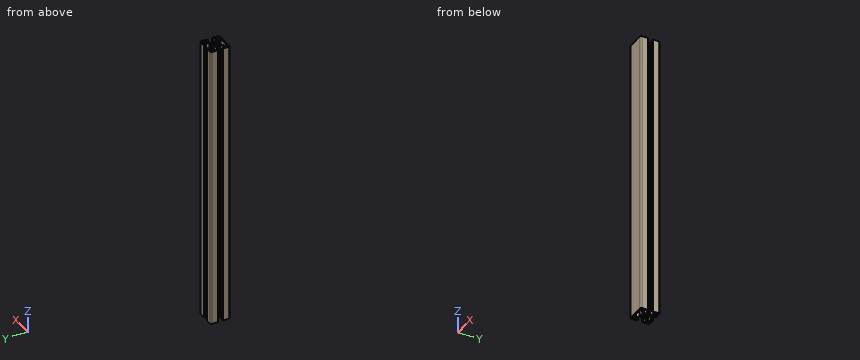
from build123d import *

# Parameters (mm, degrees)
ESTRUSIONE_ESTRUSIONE1_DEPTH = 450


with BuildPart() as part:
    # Schizzo1 → Estrusione-Estrusione1 (new body)
    with BuildSketch(Plane(origin=(0, 0, -450), x_dir=(-1, 0, 0), z_dir=(0, 0, -1))):
        with BuildLine():
            Line((-15, -4), (-15, -13))
            ThreePointArc((-15, -13), (-14.414213562, -14.414213562), (-13, -15))
            Line((-13, -15), (13, -15))
            ThreePointArc((13, -15), (14.414213562, -14.414213562), (15, -13))
            Line((15, -13), (15, -4))
            Line((15, -4), (13, -4))
            Line((13, -4), (13, -8.25))
            Line((13, -8.25), (9.664213562, -8.25))
            add(Edge.make_bspline(
                [(9.664213562, -8.25), (8.442809042, -7.028595479), (7.221404521, -5.807190958), (6, -4.585786438)],
                knots=[0, 0, 0, 0, 1, 1, 1, 1], degree=3))
            Line((6, -4.585786438), (6, -2.5))
            Line((6, -2.5), (5.750976629, -1.218885816))
            Line((5.750976629, -1.218885816), (5.933012788, -0.90358969))
            ThreePointArc((5.933012788, -0.90358969), (6, -0.653589753), (5.933012702, -0.403589838))
            Line((5.933012702, -0.403589838), (5.7, 0))
            Line((5.7, 0), (5.933012702, 0.403589838))
            ThreePointArc((5.933012702, 0.403589838), (5.982962913, 0.524180316), (6, 0.653589838))
            Line((6, 0.653589838), (6, 4.585786438))
            add(Edge.make_bspline(
                [(6, 4.585786438), (7.221404521, 5.807190958), (8.442809042, 7.028595479), (9.664213562, 8.25)],
                knots=[0, 0, 0, 0, 1, 1, 1, 1], degree=3))
            Line((9.664213562, 8.25), (13, 8.25))
            Line((13, 8.25), (13, 4))
            Line((13, 4), (15, 4))
            Line((15, 4), (15, 13))
            ThreePointArc((15, 13), (14.414213562, 14.414213562), (13, 15))
            Line((13, 15), (4, 15))
            Line((4, 15), (4, 13))
            Line((4, 13), (8.25, 13))
            Line((8.25, 13), (8.25, 9.664213562))
            add(Edge.make_bspline(
                [(8.25, 9.664213562), (7.028595479, 8.442809042), (5.807190958, 7.221404521), (4.585786438, 6)],
                knots=[0, 0, 0, 0, 1, 1, 1, 1], degree=3))
            Line((4.585786438, 6), (2.5, 6))
            Line((2.5, 6), (1.218885629, 5.750976592))
            Line((1.218885629, 5.750976592), (0.903589838, 5.933012702))
            ThreePointArc((0.903589838, 5.933012702), (0.653589838, 6), (0.403589838, 5.933012702))
            Line((0.403589838, 5.933012702), (0, 5.7))
            Line((0, 5.7), (-0.403589838, 5.933012702))
            ThreePointArc((-0.403589838, 5.933012702), (-0.524180316, 5.982962913), (-0.653589838, 6))
            Line((-0.653589838, 6), (-4.585786438, 6))
            add(Edge.make_bspline(
                [(-4.585786438, 6), (-5.807190958, 7.221404521), (-7.028595479, 8.442809042), (-8.25, 9.664213562)],
                knots=[0, 0, 0, 0, 1, 1, 1, 1], degree=3))
            Line((-8.25, 9.664213562), (-8.25, 13))
            Line((-8.25, 13), (-4, 13))
            Line((-4, 13), (-4, 15))
            Line((-4, 15), (-13, 15))
            ThreePointArc((-13, 15), (-14.414213562, 14.414213562), (-15, 13))
            Line((-15, 13), (-15, 4))
            Line((-15, 4), (-13, 4))
            Line((-13, 4), (-13, 8.25))
            Line((-13, 8.25), (-9.664213562, 8.25))
            add(Edge.make_bspline(
                [(-9.664213562, 8.25), (-8.442809042, 7.028595479), (-7.221404521, 5.807190958), (-6, 4.585786438)],
                knots=[0, 0, 0, 0, 1, 1, 1, 1], degree=3))
            Line((-6, 4.585786438), (-6, 2.5))
            Line((-6, 2.5), (-5.750976592, 1.218885629))
            Line((-5.750976592, 1.218885629), (-5.933012702, 0.903589838))
            ThreePointArc((-5.933012702, 0.903589838), (-6, 0.653589838), (-5.933012702, 0.403589838))
            Line((-5.933012702, 0.403589838), (-5.7, 0))
            Line((-5.7, 0), (-5.933012702, -0.403589838))
            ThreePointArc((-5.933012702, -0.403589838), (-5.982962913, -0.524180316), (-6, -0.653589838))
            Line((-6, -0.653589838), (-6, -4.585786438))
            add(Edge.make_bspline(
                [(-6, -4.585786438), (-7.221404521, -5.807190958), (-8.442809042, -7.028595479), (-9.664213562, -8.25)],
                knots=[0, 0, 0, 0, 1, 1, 1, 1], degree=3))
            Line((-9.664213562, -8.25), (-13, -8.25))
            Line((-13, -8.25), (-13, -4))
            Line((-13, -4), (-15, -4))
        make_face()
        with BuildLine():
            Line((12.349838066, 9.914583088), (11.34224826, 9.54785039))
            ThreePointArc((11.34224826, 9.54785039), (9.873470565, 9.873470565), (9.54785039, 11.34224826))
            Line((9.54785039, 11.34224826), (9.914583088, 12.349838066))
            ThreePointArc((9.914583088, 12.349838066), (13.043502884, 13.043502884), (12.349838066, 9.914583088))
        make_face(mode=Mode.SUBTRACT)
        with BuildLine():
            Line((-4.58, -6), (4.58, -6))
            add(Edge.make_bspline(
                [(4.58, -6), (5.73, -7.15), (6.88, -8.3), (8.03, -9.45)],
                knots=[0, 0, 0, 0, 1, 1, 1, 1], degree=3))
            Line((8.03, -9.45), (11.1, -9.45))
            Line((11.1, -9.45), (12.361944654, -9.919036981))
            ThreePointArc((12.361944654, -9.919036981), (13.194761433, -12.872897378), (10.127586207, -12.766543418))
            ThreePointArc((10.127586207, -12.766543418), (9.169403304, -12.336446483), (8.355281336, -13))
            Line((8.355281336, -13), (-8.355281336, -13))
            ThreePointArc((-8.355281336, -13), (-9.169403304, -12.336446483), (-10.127586207, -12.766543418))
            ThreePointArc((-10.127586207, -12.766543418), (-13.194761433, -12.872897378), (-12.361944654, -9.919036981))
            Line((-12.361944654, -9.919036981), (-11.1, -9.45))
            Line((-11.1, -9.45), (-8.03, -9.45))
            add(Edge.make_bspline(
                [(-8.03, -9.45), (-6.88, -8.3), (-5.73, -7.15), (-4.58, -6)],
                knots=[0, 0, 0, 0, 1, 1, 1, 1], degree=3))
        make_face(mode=Mode.SUBTRACT)
        with BuildLine():
            Line((-11.34224826, 9.54785039), (-12.349838066, 9.914583088))
            ThreePointArc((-12.349838066, 9.914583088), (-13.043502884, 13.043502884), (-9.914583088, 12.349838066))
            Line((-9.914583088, 12.349838066), (-9.54785039, 11.34224826))
            ThreePointArc((-9.54785039, 11.34224826), (-9.873470565, 9.873470565), (-11.34224826, 9.54785039))
        make_face(mode=Mode.SUBTRACT)
        with BuildLine():
            Line((4, 3.5), (4, 2))
            ThreePointArc((4, 2), (3.879005736, 1.673879391), (3.574581393, 1.505593673))
            ThreePointArc((3.574581393, 1.505593673), (3.295837094, 1.323326833), (3.251694243, 0.993219284))
            ThreePointArc((3.251694243, 0.993219284), (3.4, 0), (3.251694243, -0.993219284))
            ThreePointArc((3.251694243, -0.993219284), (3.295837094, -1.323326833), (3.574581393, -1.505593673))
            ThreePointArc((3.574581393, -1.505593673), (3.879005736, -1.673879391), (4, -2))
            Line((4, -2), (4, -3.5))
            ThreePointArc((4, -3.5), (3.853553391, -3.853553391), (3.5, -4))
            Line((3.5, -4), (2, -4))
            ThreePointArc((2, -4), (1.673879391, -3.879005736), (1.505593673, -3.574581393))
            ThreePointArc((1.505593673, -3.574581393), (1.323326833, -3.295837094), (0.993219284, -3.251694243))
            ThreePointArc((0.993219284, -3.251694243), (0, -3.4), (-0.993219284, -3.251694243))
            ThreePointArc((-0.993219284, -3.251694243), (-1.323326833, -3.295837094), (-1.505593673, -3.574581393))
            ThreePointArc((-1.505593673, -3.574581393), (-1.673879391, -3.879005736), (-2, -4))
            Line((-2, -4), (-3.5, -4))
            ThreePointArc((-3.5, -4), (-3.853553391, -3.853553391), (-4, -3.5))
            Line((-4, -3.5), (-4, -2))
            ThreePointArc((-4, -2), (-3.879005736, -1.673879391), (-3.574581393, -1.505593673))
            ThreePointArc((-3.574581393, -1.505593673), (-3.295837094, -1.323326833), (-3.251694243, -0.993219284))
            ThreePointArc((-3.251694243, -0.993219284), (-3.4, 0), (-3.251694243, 0.993219284))
            ThreePointArc((-3.251694243, 0.993219284), (-3.295837094, 1.323326833), (-3.574581393, 1.505593673))
            ThreePointArc((-3.574581393, 1.505593673), (-3.879005736, 1.673879391), (-4, 2))
            Line((-4, 2), (-4, 3.5))
            ThreePointArc((-4, 3.5), (-3.853553391, 3.853553391), (-3.5, 4))
            Line((-3.5, 4), (-2, 4))
            ThreePointArc((-2, 4), (-1.673879391, 3.879005736), (-1.505593673, 3.574581393))
            ThreePointArc((-1.505593673, 3.574581393), (-1.323326833, 3.295837094), (-0.993219284, 3.251694243))
            ThreePointArc((-0.993219284, 3.251694243), (0, 3.4), (0.993219284, 3.251694243))
            ThreePointArc((0.993219284, 3.251694243), (1.323326833, 3.295837094), (1.505593673, 3.574581393))
            ThreePointArc((1.505593673, 3.574581393), (1.673879391, 3.879005736), (2, 4))
            Line((2, 4), (3.5, 4))
            ThreePointArc((3.5, 4), (3.853553391, 3.853553391), (4, 3.5))
        make_face(mode=Mode.SUBTRACT)
    extrude(amount=-ESTRUSIONE_ESTRUSIONE1_DEPTH)


solid = part.part
Can you work these out from the model? Positions are in its coordinate system, mm. Give positions to 0.01 mm unless a question says otherwise; leave off trailing zeros. Answer as a JSON object with one key per item and string values.
Q1. Will these pins go through, and if not, where does the flat tip stop? P1, Ø1.6, axis at x = 2.5, z = -306.5, coming from the +Y side; P2, Ø0.8, axis at y = 2.5, z = -187.5, coming from the +X side; P3, Ø1.6, axis at x = -14, z = -279, coming from the -Y side.
Geometry says:
{"P1": "y = 6", "P2": "x = 6", "P3": "y = -14.99"}
Q2. If I drill on L1, parallel to Y at x = 11.7, z = -279; L2, parallel to X at y = 11.7, z = -223; L3, parallel to Y at x = 1, z = -47.5, over which ranges is the centre line in solid material (lowest first)?
Geometry says:
{"L1": "-15 to -13.6, -9.67 to -8.25, 8.25 to 9.68, 13.6 to 15", "L2": "-15 to -13.6, -9.68 to -8.25, 8.25 to 9.68, 13.6 to 15", "L3": "-15 to -13, -6 to -3.25, 3.25 to 6"}
Q3. Imagine slicing it at A-A on z = -43. Give the number of separate pieces and of enclosed holes in the cut face, plus the area to 3 significant figures.
Geometry says:
{"separate pieces": "1", "enclosed holes": "4", "area": "323 mm²"}
